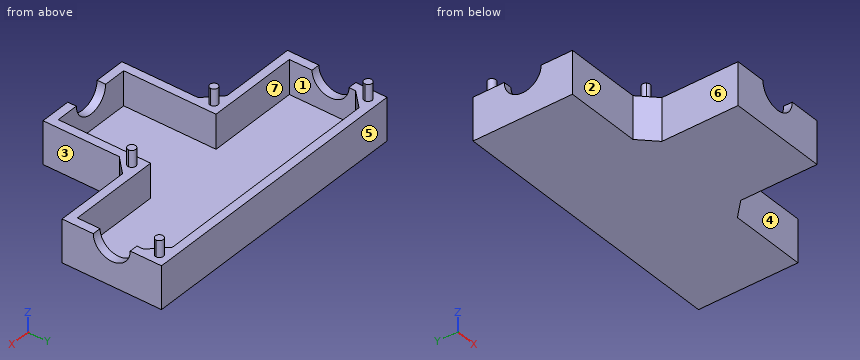
```python
from build123d import *

# Parameters (mm, degrees)
F1_DEPTH  = 7.5
F2_T      = -1.5
F4_DEPTH  = 7.5
F6_DEPTH  = 2.9
F7_R      = 3.25
F8_DEPTH  = 32.25
F9_R      = 3.25
F10_DEPTH = 50.001


with BuildPart() as f1:
    # F0 (on Top) → F1 (new body)
    with BuildSketch(Plane.XY):
        Polygon((25, -8.75), (25, 8.75), (8.75, 8.75), (-8.75, 8.75), (-25, 8.75), (-25, -8.75), (-8.75, -8.75), (-8.75, -25), (0, -25), (8.75, -25), (8.75, -8.75), align=None)
    extrude(amount=F1_DEPTH)

    # F2
    f2_openings = [f1.faces().sort_by_distance(p)[0] for p in [
        (0, -4.139151, 7.5),
    ]]
    offset(amount=F2_T, openings=f2_openings, kind=Kind.INTERSECTION)

    # F3 (on face) → F4 (join, through all)
    with BuildSketch(Plane.XY.offset(7.5)):
        Polygon((-23.5, 7.25), (-23.5, 4.4215728753), (-20.6715728753, 7.25), align=None)
        Polygon((-8.75, -8.75), (-11.5784271247, -8.75), (-8.75, -11.5784271247), align=None)
        Polygon((23.5, 7.25), (20.6715728753, 7.25), (23.5, 4.4215728753), align=None)
        Polygon((8.75, -11.5784271247), (11.5784271247, -8.75), (8.75, -8.75), align=None)
    extrude(amount=-F4_DEPTH)

    # F5 (on face) → F6 (join)
    with BuildSketch(Plane.XY.offset(7.5)):
        with BuildLine():
            ThreePointArc((-9.5985281374, -9.5985281374), (-8.8356749879, -9.7502690634), (-8.4035533906, -9.1035533906))
            ThreePointArc((-8.4035533906, -9.1035533906), (-9.3714317932, -8.4568377178), (-9.5985281374, -9.5985281374))
        make_face()
        with BuildLine():
            ThreePointArc((-22.6514718626, 6.4014718626), (-22.4997309366, 6.6285682068), (-22.4464466094, 6.8964466094))
            ThreePointArc((-22.4464466094, 6.8964466094), (-23.7931622822, 7.1643250121), (-22.6514718626, 6.4014718626))
        make_face()
        with BuildLine():
            ThreePointArc((9.5985281374, -9.5985281374), (9.7502690634, -9.3714317932), (9.8035533906, -9.1035533906))
            ThreePointArc((9.8035533906, -9.1035533906), (8.4568377178, -8.8356749879), (9.5985281374, -9.5985281374))
        make_face()
        with BuildLine():
            ThreePointArc((22.6514718626, 6.4014718626), (23.4143250121, 6.2497309366), (23.8464466094, 6.8964466094))
            ThreePointArc((23.8464466094, 6.8964466094), (22.8785682068, 7.5431622822), (22.6514718626, 6.4014718626))
        make_face()
    extrude(amount=F6_DEPTH)

    # F7 (on face) → F8 (cut, through all)
    with BuildSketch(Plane.XZ.offset(25)):
        with Locations((0, 7.5)):
            Circle(F7_R)
    extrude(amount=-F8_DEPTH, mode=Mode.SUBTRACT)

    # F9 (on face) → F10 (cut, through all)
    with BuildSketch(Plane(origin=(-25, 0, 0), x_dir=(0, -1, 0), z_dir=(-1, 0, 0))):
        with Locations((0, 7.5)):
            Circle(F9_R)
    extrude(amount=-F10_DEPTH, mode=Mode.SUBTRACT)


solid = f1.part
```
Check sheet for the modelled part. Datum: model origin and axes. Units: mm. Face numbers are marked on the shaded views. A direction names the side the tool comes from. Give positions to 0.01 mm unless a question says otherwise; leave off trailing zeros. Order: outer loops, then holes, each group sorted by start corner. A loop starts at its lowest first (then second) coordinate and runs counter-clockwise, first axis right, second up. Notation, with made-up numbers: (62, 31) -> (92, 31) arc R29 cw to (92, 68) -> close; hole circle Ø9 at (42.25, 69). An arc over 180 degrees is marked (long way). Return JSON: item names as keys, results as strings.
1. Material ranges on probe 1 along Y at (x, z) = (20, 3.5); probe 2 along Y at (x, z) = (-5, 2.25), recorded low to high. Write a range as [from, to].
From the geometry:
{"probe 1": "[-8.75, -7.25], [7.25, 8.75]", "probe 2": "[-25, -23.5], [7.25, 8.75]"}
2. Go/stop test with flat-tipped pins: P1, Ø4, axis at y = -14, z = 9, coming from the +X side; P2, Ø5, axis at x = -2, z = 9, coming from the -Y side; P3, Ø4, axis at y = -15.5, z = 3.5, coming from the -X side; P4, Ø3, axis at y = -12, z = 3, coming from the -X side. Record where each tip stops, or that it passes through.
From the geometry:
{"P1": "x = 8.75", "P2": "y = -25", "P3": "x = -8.75", "P4": "x = -9.83"}
3. Set-up check for the marked faces 1, 2 and 3: record each of +Z, -Z, +X, -X, +Y, -Y from which the full face is reachable in a straight line by a thin tool's end or side.
From the geometry:
{"face 1": "+Z", "face 2": "+Z, -Z, -X, -Y", "face 3": "+Z, -Z, +X, -Y"}
4. Cross-section at B-B, the plane x = 0. Record the cut outline in (y, z), plus the area to 4 significant figures.
From the geometry:
{"outline": "(-25, 0) -> (8.75, 0) -> (8.75, 7.5) -> (7.25, 7.5) -> (7.25, 1.5) -> (-23.5, 1.5) -> (-23.5, 4.25) -> (-25, 4.25) -> close", "area": "63.75 mm^2"}
5. Cross-section at C-C, the plane y = 0. Record the cut outline in (x, z), plus the area to 4 significant figures.
From the geometry:
{"outline": "(-25, 0) -> (25, 0) -> (25, 4.25) -> (23.5, 4.25) -> (23.5, 1.5) -> (-23.5, 1.5) -> (-23.5, 4.25) -> (-25, 4.25) -> close", "area": "83.25 mm^2"}
6. Mould release check, pull along Y, two halves, no side actions. Record for the marked faces 4, 5, 6 and 7: +Y half, -Y half, draft (parallel to the pull), parting line (faces both ways), or undercut.
From the geometry:
{"face 4": "-Y half", "face 5": "+Y half", "face 6": "draft", "face 7": "undercut"}
7. Cross-section at A-A, the plane z = 2. Record the cut outline in (x, y).
From the geometry:
{"outline": "(-25, -8.75) -> (-11.58, -8.75) -> (-8.75, -11.58) -> (-8.75, -25) -> (8.75, -25) -> (8.75, -11.58) -> (11.58, -8.75) -> (25, -8.75) -> (25, 8.75) -> (-25, 8.75) -> close; hole (-23.5, -7.25) -> (-7.25, -7.25) -> (-7.25, -23.5) -> (7.25, -23.5) -> (7.25, -7.25) -> (23.5, -7.25) -> (23.5, 4.42) -> (20.67, 7.25) -> (-20.67, 7.25) -> (-23.5, 4.42) -> close"}
8. Cross-section at D-D, the plane z = 8. Record the cut outline in (x, y), plus the area to 3 significant figures.
From the geometry:
{"outline": "circle Ø1.4 at (-23.15, 6.9); circle Ø1.4 at (-9.1, -9.1); circle Ø1.4 at (9.1, -9.1); circle Ø1.4 at (23.15, 6.9)", "area": "6.16 mm^2"}
